Verification items for the finished model (mm, model axes). A direction names the side the tool comes from. Give positions to 0.01 mm unless a question says otherwise; leave off trailing zeros. Order: outer loops, then holes, each group sorted by start corner. A loop starts at its lowest first (then second) coordinate and runs counter-clockwise, first axis right, second up. Notation, with made-up numbers: M 47,-20 L 79,-20 A29 ccw 79,14 Z; hole C -28.5,73 d2. An arc over 180 degrees is marked long. Answer as a JSON object with one key per item and string values.
```python
from build123d import *

# Parameters (mm, degrees)
BOSS_EXTRUDE1_DEPTH = 65.8876
BOSS_EXTRUDE2_DEPTH = 29.3624
BOSS_EXTRUDE3_DEPTH = 2.54
SKETCH4_R           = 2
BOSS_EXTRUDE4_DEPTH = 2.54
SKETCH6_W           = 24.561
SKETCH6_H           = 12.2809
BOSS_EXTRUDE5_DEPTH = 2.54
CUT_EXTRUDE1_DEPTH  = 101.281127945
FILLET1_R           = 1.27
FILLET2_R           = 1.27
FILLET4_R           = 1.27
SKETCH8_R           = 3.8
SKETCH8_R_2         = 3.80000002
CUT_EXTRUDE2_DEPTH  = 12.9159


with BuildPart() as part:
    # Sketch1 → Boss-Extrude1 (new body)
    with BuildSketch(Plane(origin=(0, 0, 0), x_dir=(0, 0, -1), z_dir=(1, 0, 0))):
        with BuildLine():
            Line((34.207401555, 10.336569156), (37.382401555, 10.336569156))
            Line((37.382401555, 10.336569156), (37.382401555, -5.119330844))
            Line((37.382401555, -5.119330844), (21.926501555, -5.119330844))
            Line((21.926501555, -5.119330844), (21.926501555, -1.944330844))
            ThreePointArc((21.926501555, -1.944330844), (30.610409224, 1.652661487), (34.207401555, 10.336569156))
        make_face()
    extrude(amount=BOSS_EXTRUDE1_DEPTH)

    # Sketch2 → Boss-Extrude2 (add)
    with BuildSketch(Plane(origin=(65.8876, 0, 0), x_dir=(0, 0, -1), z_dir=(1, 0, 0))):
        Polygon((37.382401555, -1.944330844), (37.382401555, 10.336569156), (34.207401555, 10.336569156), (34.207401555, -1.944330844), (9.646401555, -1.944330844), (9.646401555, -5.119330844), (37.382401555, -5.119330844), align=None)
    boss_extrude2 = extrude(amount=BOSS_EXTRUDE2_DEPTH)

    # Sketch3 → Boss-Extrude3 (add)
    with BuildSketch(Plane(origin=(95.25, 0, 0), x_dir=(0, 0, -1), z_dir=(1, 0, 0))):
        Polygon((28.207401555, 4.196119156), (13.646401555, 4.196119156), (13.646401555, 10.336569156), (9.646401555, 10.336569156), (9.646401555, 4.196119156), (9.646401555, -1.944330844), (28.207401555, -1.944330844), (34.207401555, -1.944330844), (34.207401555, 10.336569156), (28.207401555, 10.336569156), align=None)
    extrude(amount=-BOSS_EXTRUDE3_DEPTH)

    # Sketch4 → Boss-Extrude4 (add)
    # profile 1 of 3: a face of its own
    with BuildSketch(Plane.XY.offset(-21.926501555)):
        with BuildLine():
            Line((0, -8.294330844), (0, -5.119330844))
            Line((0, -5.119330844), (12.7, -5.119330844))
            Line((12.7, -5.119330844), (12.7, -8.294330844))
            ThreePointArc((12.7, -8.294330844), (6.35, -14.644330844), (0, -8.294330844))
        make_face()
        with Locations((6.35, -8.294330844)):
            Circle(SKETCH4_R, mode=Mode.SUBTRACT)
    # profile 2 of 3: a face of its own
    with BuildSketch(Plane.XY.offset(-21.926501555)):
        with BuildLine():
            Line((26.5938, -8.294330844), (26.5938, -5.119330844))
            Line((26.5938, -5.119330844), (39.2938, -5.119330844))
            Line((39.2938, -5.119330844), (39.2938, -8.294330844))
            ThreePointArc((39.2938, -8.294330844), (32.9438, -14.644330844), (26.5938, -8.294330844))
        make_face()
        with Locations((32.9438, -8.294330844)):
            Circle(SKETCH4_R, mode=Mode.SUBTRACT)
    # profile 3 of 3: a face of its own
    with BuildSketch(Plane.XY.offset(-21.926501555)):
        with BuildLine():
            Line((53.1876, -5.119330844), (65.8876, -5.119330844))
            Line((65.8876, -5.119330844), (65.8876, -8.294330844))
            ThreePointArc((65.8876, -8.294330844), (59.5376, -14.644330844), (53.1876, -8.294330844))
            Line((53.1876, -8.294330844), (53.1876, -5.119330844))
        make_face()
        with Locations(Location((59.5376, -8.294330844, 0), (0, 0, 180))):
            Circle(SKETCH4_R, mode=Mode.SUBTRACT)
    extrude(amount=-BOSS_EXTRUDE4_DEPTH)

    # Mirror1: Boss-Extrude2 across plane
    add(boss_extrude2.mirror(Plane(origin=(32.9438, 0, 0), x_dir=(0, 0, 1), z_dir=(1, 0, 0))))

    # Sketch6 → Boss-Extrude5 (add)
    with BuildSketch(Plane.ZY.offset(29.3624)):
        with Locations((-21.926901555, 4.196119156)):
            Rectangle(SKETCH6_W, SKETCH6_H)
    extrude(amount=-BOSS_EXTRUDE5_DEPTH)

    # Sketch7 → Cut-Extrude1 (cut, through all)
    with BuildSketch(Plane(origin=(0, 0, -37.382401555), x_dir=(-1, 0, 0), z_dir=(0, 0, -1))):
        Polygon((4.19354, 9.257069156), (4.19354, 10.336569156), (21.209, 10.336569156), (21.209, 9.257069156), (21.209, 5.066069156), (4.19354, 5.066069156), align=None)
    extrude(amount=-CUT_EXTRUDE1_DEPTH, mode=Mode.SUBTRACT)

    # Fillet1
    fillet1_edges = [part.edges().sort_by_distance(p)[0] for p in [
        (-29.3624, -5.119330844, -23.514401555),
        (-29.3624, 10.336569156, -23.514401555),
        (95.25, -5.119330844, -23.514401555),
    ]]
    fillet(fillet1_edges, radius=FILLET1_R)

    # Fillet2
    fillet2_edges = [part.edges().sort_by_distance(p)[0] for p in [
        (0, -5.119330844, -23.196501555),
        (12.7, -5.119330844, -23.196501555),
        (26.5938, -5.119330844, -23.196501555),
        (39.2938, -5.119330844, -23.196501555),
        (65.8876, -5.119330844, -23.196501555),
        (53.1876, -5.119330844, -23.196501555),
    ]]
    fillet(fillet2_edges, radius=FILLET2_R)

    # Fillet4
    fillet4_edges = [part.edges().sort_by_distance(p)[0] for p in [
        (-26.8224, -1.944330844, -21.926901555),
        (92.71, -1.944330844, -21.926901555),
    ]]
    fillet(fillet4_edges, radius=FILLET4_R)

    # Sketch8 → Cut-Extrude2 (cut)
    with BuildSketch(Plane(origin=(0, 0, -37.382401555), x_dir=(-1, 0, 0), z_dir=(0, 0, -1))):
        with Locations((-59.5376, -8.294330844)):
            Circle(SKETCH8_R)
        with Locations((-32.9438, -8.294330844)):
            Circle(SKETCH8_R_2)
        with Locations((-6.35, -8.294330844)):
            Circle(SKETCH8_R_2)
    extrude(amount=-CUT_EXTRUDE2_DEPTH, mode=Mode.SUBTRACT)


solid = part.part
```
Q1. Gauge pin test, flat ends, axial feed: pin 1 Ø4.5 at (x, y) = (6.35, -8.29) entering from -Z; pin 2 Ø7.5 at (x, z) = (18, -30) entering from -Y; pin 3 Ø14 at (x, y) = (25, -8.5) entering from +Z. Record the tip position at first contact, or that the pin passes through.
Resolved:
{"pin 1": "stops at z = -24.47", "pin 2": "stops at y = -5.12", "pin 3": "stops at z = -21.93"}
Q2. Material ranges on L1, parallel to X at y = 0.5, z = -31.5; L2, parallel to X at y = 6.5, z = -32; L3, parallel to Y at x = 77, z = -36, recorded low to high.
Resolved:
{"L1": "x = -29.36 to -26.82, 0 to 65.89, 92.71 to 95.25", "L2": "x = -29.36 to -26.82, 92.71 to 95.25", "L3": "y = -5.12 to 10.34"}
Q3. Release check for a two-part mould opening along X. For faces 6 (the face through (95.25, 2, -23)), 7 (the face through (92.71, 4, -22)), 8 (the face through (94, 7, -28.207)) record: +X half, -X half, draft (parallel to the pull), parting line (faces both ways), or undercut.
Resolved:
{"face 6": "+X half", "face 7": "undercut", "face 8": "draft"}
Q4. Tool access check on faces 1 (the face through (59.677, -14.643, -23.179)), 2 (the face through (-26.822, 5, -22)), 3 (the face through (-21.209, 8, -36)), 4 (the face through (-18, -3, -9.646)), 5 (the face through (46, -5.119, -30)). Record the directions out of +Z, -Z, +X, -X, +Y, -Y that give a thin tool (end or side, any length) a straight path to the whole face; none if there is none.
Resolved:
{"face 1": "+Z, -Z, -Y", "face 2": "+Z, +Y", "face 3": "+Z, -Z, +Y", "face 4": "+Z, +X, -X, +Y, -Y", "face 5": "-Z, -Y"}
Q5. Section check D-D on x = 22.5. Record the cut outline in (y, z).
Resolved:
{"outline": "M -5.12,-37.38 L 10.34,-37.38 L 10.34,-34.21 A12.28 cw -1.94,-21.93 L -5.12,-21.93 Z"}
Q6. Section check C-C on y = 6.5. Record the cut outline in (x, z), then the cut area to 3 significant figures.
Resolved:
{"outline": "M -29.36,-37.38 L -21.21,-37.38 L -21.21,-34.21 L -26.82,-34.21 L -26.82,-9.65 L -29.36,-9.65 Z; M -4.19,-37.38 L 95.25,-37.38 L 95.25,-28.21 L 92.71,-28.21 L 92.71,-34.21 L 65.89,-34.21 L 65.89,-33.59 L 0,-33.59 L 0,-34.21 L -4.19,-34.21 Z; M 92.71,-13.65 L 95.25,-13.65 L 95.25,-9.65 L 92.71,-9.65 Z", "area": "470 mm²"}
Q7. Section check A-A on x = 6.35. Record the cut outline in (y, z), then the cut area to 3 significant figures.
Resolved:
{"outline": "M -14.64,-24.47 L -10.29,-24.47 L -10.29,-21.93 L -14.64,-21.93 Z; M -6.29,-24.47 L -4.49,-24.47 L -4.49,-37.38 L 10.34,-37.38 L 10.34,-34.21 A12.28 cw -1.94,-21.93 L -6.29,-21.93 Z", "area": "126 mm²"}
Q8. Section check B-B on z = -20.5. Record the cut outline in (x, y), then the cut area to 3 significant figures.
Resolved:
{"outline": "M -29.36,-3.85 A1.27 ccw -28.09,-5.12 L 0,-5.12 L 0,-1.94 L -25.55,-1.94 A1.27 cw -26.82,-0.67 L -26.82,10.34 L -28.09,10.34 A1.27 ccw -29.36,9.07 Z; M 65.89,-5.12 L 93.98,-5.12 A1.27 ccw 95.25,-3.85 L 95.25,4.2 L 92.71,4.2 L 92.71,-0.67 A1.27 cw 91.44,-1.94 L 65.89,-1.94 Z", "area": "233 mm²"}
